Verification items for the finished model (mm, model axes). A direction names the side the tool comes from. Give positions to 0.01 mm unless a question says otherwise; leave off trailing zeros. Loops run counter-clockwise (first coordinate to the right, second up) from the corner with the lowest first, then second, coordinate; pieces in that order, holes last. Notation, with made-up numbers: (45.5, 12) -> (62.5, 12) arc R29 cw to (62.5, 40) -> close; hole circle Ø8 at (71, -10). An arc over 180 degrees is marked (long way). Answer in a Markdown table with one row per item. Add a question column.
Q1. Section check D-D on z = 7.25. Enter the section's corners in (x, y).
Q2. Release check for a two-part mould opening along X. For faces 1 (the face through (5.8, 9.7, 21.9)), 2 (the face through (4.96, -2.96, 15.81)), 3 (the face through (6, 17, 27.5)) record: pulls with the +X half, pulls with the -X half, needs draft (parallel to the pull), parting line crosses it, or undercut.
Q3. Set-up check for faces 4 (the face through (6, 24, 15)), 5 (the face through (6, -1, 15)), 6 (the face through (4, 25, 16.6)), 7 (the face through (1, 22, 19.65)): record each of +Z, -Z, +X, -X, +Y, -Y from which the full face is reachable in a straight line by a thin tool's end or side.
Q4. Section check B-B on x = 5.25. Give the number of separate pieces and of enclosed holes in the cut face, and give its area (3 significant figures).
Q5. Section check A-A on y = -2.35. Enter the section's corners in (x, z), and give its area (3 significant figures).
Q6. Material ranges on probe 1 along Y at (x, z) = (5.75, 15.45); probe 2 along Z at (x, y) = (8.25, 14.5); probe 3 along Y at (x, z) = (5.25, 12), recorded low to high.
Q7. Gauge pin test, flat ends, axial feed: P1, Ø3, axis at x = 5.75, y = -2.35, coming from the +Z side; P2, Ø1.5, axis at x = 3.5, z = 18, coming from the -Y side; P3, Ø5, axis at x = 1.5, y = 10.5, coming from the +Z side. Record the tip position at first contact, or that the pin passes through.
Q8. Section check C-C on x = 10. Enter the section's corners in (y, z).
```python
from build123d import *

# Parameters (mm, degrees)
F1_DEPTH = 11.5
F3_DEPTH = 4.35
F4_R     = 5
F5_R     = 1
F6_DEPTH = 25
F7_R     = 2
F8_DEPTH = 3.5


with BuildPart() as f1:
    # F0 (on Right) → F1 (new body)
    with BuildSketch(Plane.YZ):
        Polygon((0, 15), (0, 0), (18.8086195217, 0), (23, 2.3149361368), (23, 15), (27.5, 15), (27.5, 16.6), (23, 16.6), (23, 24), (5, 24), (5, 19.65), (0, 19.65), (0, 16.6), (-4.5, 16.6), (-4.5, 15), align=None)
    extrude(amount=F1_DEPTH)

    # F2 (on face) → F3 (cut, through all)
    with BuildSketch(Plane.XY.offset(24)):
        with BuildLine():
            Line((11.5, 5), (11.5, 17.25))
            ThreePointArc((11.5, 17.25), (10.4021463443, 13.8706458618), (7.5278141248, 11.7817391304))
            ThreePointArc((7.5278141248, 11.7817391304), (7.5444449594, 11.6413056534), (7.55, 11.5))
            ThreePointArc((7.55, 11.5), (5.6086943466, 9.7055550406), (3.9721858752, 11.7817391304))
            ThreePointArc((3.9721858752, 11.7817391304), (1.0978536557, 13.8706458618), (0, 17.25))
            Line((0, 17.25), (0, 5))
            Line((0, 5), (11.5, 5))
        make_face()
        with BuildLine():
            ThreePointArc((5.75, 23), (9.8158639918, 21.3158639918), (11.5, 17.25))
            Line((11.5, 17.25), (11.5, 23))
            Line((11.5, 23), (5.75, 23))
        make_face()
        with BuildLine():
            ThreePointArc((0, 17.25), (1.6841360082, 21.3158639918), (5.75, 23))
            Line((5.75, 23), (0, 23))
            Line((0, 23), (0, 17.25))
        make_face()
    extrude(amount=-F3_DEPTH, mode=Mode.SUBTRACT)

    # F4
    f4_edges = [f1.edges().sort_by_distance(p)[0] for p in [
        (7.527814, 11.781739, 21.825),
        (3.972186, 11.781739, 21.825),
    ]]
    fillet(f4_edges, radius=F4_R)

    # F5 (on face) → F6 (cut)
    with BuildSketch(Plane.XY.offset(16.6)):
        with BuildLine():
            ThreePointArc((5.75, 24.25), (6.4571067812, 24.5428932188), (6.75, 25.25))
            ThreePointArc((6.75, 25.25), (6.4571067812, 25.9571067812), (5.75, 26.25))
            Line((5.75, 26.25), (5.75, 24.25))
        make_face()
        with BuildLine():
            Line((5.75, 24.25), (5.75, 26.25))
            ThreePointArc((5.75, 26.25), (4.75, 25.25), (5.75, 24.25))
        make_face()
        with Locations((5.75, -2.35)):
            Circle(F5_R)
    extrude(amount=-F6_DEPTH, mode=Mode.SUBTRACT)

    # F7 (on face) → F8 (join)
    with BuildSketch(Plane.XY.offset(24)):
        with Locations((5.75, 17.25)):
            Circle(F7_R)
    extrude(amount=F8_DEPTH)


solid = f1.part
```
Taken from the geometry:
| question | item | result |
|---|---|---|
| 1 | outline | (0, 0) -> (11.5, 0) -> (11.5, 23) -> (0, 23) -> close |
| 2 | face 1 | parting line crosses it |
| 2 | face 2 | undercut |
| 2 | face 3 | needs draft |
| 3 | face 4 | -Z, +X, -X, +Y |
| 3 | face 5 | -Z, +X, -X, -Y |
| 3 | face 6 | +Z, +X, -X, +Y |
| 3 | face 7 | +Z, -X, +Y |
| 4 | separate pieces | 3 |
| 4 | enclosed holes | 0 |
| 4 | area | 527 mm² |
| 5 | outline | (0, 15) -> (4.75, 15) -> (4.75, 16.6) -> (0, 16.6) -> close; (6.75, 15) -> (11.5, 15) -> (11.5, 16.6) -> (6.75, 16.6) -> close |
| 5 | area | 15.2 mm² |
| 6 | probe 1 | y = -4.5 to -3.35, -1.35 to 24.25, 26.25 to 27.5 |
| 6 | probe 2 | z = 0 to 24 |
| 6 | probe 3 | y = 0 to 23 |
| 7 | P1 | stops at z = 16.6 |
| 7 | P2 | stops at y = 0 |
| 7 | P3 | stops at z = 24 |
| 8 | outline | (-4.5, 15) -> (0, 15) -> (0, 0) -> (18.81, 0) -> (23, 2.31) -> (23, 15) -> (27.5, 15) -> (27.5, 16.6) -> (23, 16.6) -> (23, 19.65) -> (21.12, 19.65) -> (21.12, 24) -> (13.38, 24) -> (13.38, 19.65) -> (0, 19.65) -> (0, 16.6) -> (-4.5, 16.6) -> close |
